Read the model definition and answer for the solid it produces. Units are mm, in the model's axes. A direction names the side the tool comes from. Give positions to 0.01 mm unless a question says otherwise; leave off trailing zeros. Loops run counter-clockwise (first coordinate to the right, second up) from the corner with the lowest first, then second, coordinate; pieces in that order, holes last.
(1) Find section C-C, the plane x = 0. Write down the section's boundary in (y, z), then the cut area to 3 significant figures.
(2) Which of the six approach directions +Z, -Z, +X, -X, +Y, -Y give full straight-line access (tool end or side, diameter ignored) to faces 5 (the face through (10.409, -7, 0)), 6 (the face through (10, -7, 1.945)), 7 (the face through (-2, -15, 0)), 8 (the face through (10, -7, -1.855)), 9 (the face through (1.5, -9, 0))?
(3) Find section D-D, the plane x = 9.25. Write down the section's boundary in (y, z).
(4) Find section A-A, the plane y = -11.25. Write down the section's boundary in (x, z), then the cut area to 3 significant figures.
(5) Find section B-B, the plane z = 3.5. Write down the section's boundary in (x, y), then the cut area to 3 significant figures.
(6) Each of these flat-tipped pins is pushed along its axis until it touches: P1, Ø3, axis at y = -7.5, z = -3.5, coming from the +X side; P2, Ø1.5, axis at x = -0.5, z = 2.5, coming from the -Y side; P3, Ø0.6, axis at x = -2.5, y = -5.5, coming from the -Z side. Where does it stop, or does it pass through?
(7) Determine the mould class of faces 1 (the face through (-9.094, -7.395, 0.327)), 2 (the face through (0, -9, 7)), 3 (the face through (1, 0, 0)), 4 (the face through (-2, -9, -3.809)) for opening direction Z: pulls with the +Z half, pulls with the -Z half, needs draft (parallel to the pull), parting line crosses it, or undercut.
(8) Straight lines are drawn through the part: probe 1 along Z at (x, y) = (1, -5.5); probe 2 along X at (y, z) = (-4.5, 2); probe 3 along X at (y, z) = (-13, 3.25). For each, find the intervals that lie inside material, in ascending order.
```python
from build123d import *

# Parameters (mm, degrees)
PAD_DEPTH    = 15
POCKET_DEPTH = 13


with BuildPart() as part:
    # Sketch → Pad (new body)
    with BuildSketch(Plane.XZ):
        with BuildLine():
            ThreePointArc((8.889624, 1.945402), (-9.099882, -0.046426), (8.90901, -1.854598))
            Line((10.40901, -1.854598), (8.90901, -1.854598))
            Line((10.40901, 1.945402), (10.40901, -1.854598))
            Line((8.889624, 1.945402), (10.40901, 1.945402))
        make_face()
    extrude(amount=PAD_DEPTH)

    # Sketch001 (on Face6 of Pad) → Pocket (cut)
    with BuildSketch(Plane.XZ.offset(15)):
        Polygon((-1.5, 7), (1.5, 7), (1.5, -7), (-3.348355, -7), (-3.348355, -3.808815), (-1.5, -3.808815), align=None)
    extrude(amount=-POCKET_DEPTH, mode=Mode.SUBTRACT)


solid = part.part
```
Entries:
1. outline: (-15, -9.1) - (0, -9.1) - (0, 9.1) - (-15, 9.1) - (-15, 7) - (-2, 7) - (-2, -7) - (-15, -7) - close
1. area: 91.0 mm2
2. face 5: +Z, -Z, +X, +Y, -Y
2. face 6: +Z, +X, +Y, -Y
2. face 7: +Z, -Z, +X, -X, -Y
2. face 8: -Z, +X, +Y, -Y
2. face 9: -Y
3. outline: (-15, -1.85) - (0, -1.85) - (0, 1.95) - (-15, 1.95) - close
4. outline: (8.89, 1.95) arc R9.1 ccw (long way) to (8.91, -1.85) - (10.41, -1.85) - (10.41, 1.95) - close; hole (-3.35, -7) - (1.5, -7) - (1.5, 7) - (-1.5, 7) - (-1.5, -3.81) - (-3.35, -3.81) - close
4. area: 217 mm2
5. outline: (-8.4, -15) - (-1.5, -15) - (-1.5, -2) - (1.5, -2) - (1.5, -15) - (8.4, -15) - (8.4, 0) - (-8.4, 0) - close
5. area: 213 mm2
6. P1: stops at x = 8.88
6. P2: stops at y = -2
6. P3: stops at z = -8.83
7. face 1: parting line crosses it
7. face 2: undercut
7. face 3: needs draft
7. face 4: undercut
8. probe 1: z = -9.04 to -7, 7 to 9.04
8. probe 2: x = -8.88 to -1.5, 1.5 to 8.88
8. probe 3: x = -8.5 to -1.5, 1.5 to 8.5
